Check sheet for the modelled part. Datum: model origin and axes. Units: mm. Give positions to 0.01 mm unless a question says otherwise; leave off trailing zeros. Write each loop counter-clockwise with the first axis right and the second up, starting at its lowest first coordinate (ties: lowest second). Pieces come first, ordered by that corner, then holes. Notation, with made-up numbers: (51.5, 80) -> (98.5, 80) arc R24 cw to (98.5, 104) -> close; hole circle Ø9 at (57, 17.25). An arc over 180 degrees is marked (long way). Return JSON: item names as keys, results as strings.
from build123d import *

# Parameters (mm, degrees)
BOSS_EXTRUDE1_DEPTH = 10
SKETCH2_W           = 40.182856857
SKETCH2_H           = 10
BOSS_EXTRUDE2_DEPTH = 10


with BuildPart() as part:
    # Sketch1 → Boss-Extrude1 (new body)
    with BuildSketch(Plane(origin=(0, 0, 0), x_dir=(1, 0, 0), z_dir=(0, 1, 0))):
        with BuildLine():
            Line((137, 124), (0, 124))
            Line((0, 124), (0, 0))
            Line((0, 0), (137, 0))
            Line((137, 0), (137, 12))
            Line((137, 12), (111.1, 12))
            ThreePointArc((111.1, 12), (59.1, 64), (111.1, 116))
            Line((111.1, 116), (137, 116))
            Line((137, 116), (137, 124))
        make_face()
    extrude(amount=BOSS_EXTRUDE1_DEPTH)

    # Sketch2 → Boss-Extrude2 (add)
    with BuildSketch(Plane(origin=(0, 10, 0), x_dir=(1, 0, 0), z_dir=(0, 1, 0))):
        with Locations((116.908571572, 119)):
            Rectangle(SKETCH2_W, SKETCH2_H)
    extrude(amount=-BOSS_EXTRUDE2_DEPTH)


solid = part.part
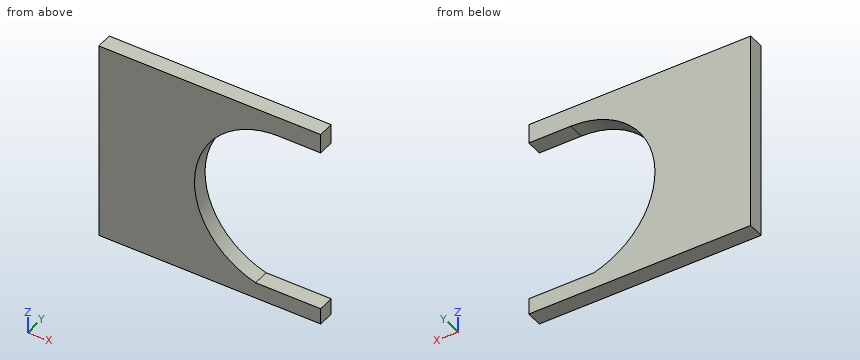
(1) Cross-section at C-C on x = 89. Enter the section's corners in (y, z).
Reply:
{"outline": "(0, -124) -> (10, -124) -> (10, -111.07) -> (0, -111.07) -> close; (0, -16.93) -> (10, -16.93) -> (10, 0) -> (0, 0) -> close"}
(2) Cross-section at D-D on z = -105.5. Enter the section's corners in (x, y), then the cut area to 3 significant figures.
Reply:
{"outline": "(0, 0) -> (79.77, 0) -> (79.77, 10) -> (0, 10) -> close", "area": "798 mm^2"}
(3) Cross-section at A-A on x = 121. Enter the section's corners in (y, z), then the cut area to 3 significant figures.
Reply:
{"outline": "(0, -124) -> (10, -124) -> (10, -114) -> (0, -114) -> close; (0, -12) -> (10, -12) -> (10, 0) -> (0, 0) -> close", "area": "220 mm^2"}
(4) Cross-section at B-B on y = 6.5. Enter the section's corners in (x, z).
Reply:
{"outline": "(0, -124) -> (137, -124) -> (137, -114) -> (96.82, -114) arc R52 cw to (111.1, -12) -> (137, -12) -> (137, 0) -> (0, 0) -> close"}
(5) Depth check by flat-ended pin: pin 1 Ø6 at (y, z) = (7.5, -56) entering from +X; pin 2 Ø4 at (y, z) = (3, -39) entering from +X; pin 3 Ø6 at (y, z) = (7, -108) entering from +X. Enter the tip coordinate at first touch or a pass-through.
Reply:
{"pin 1": "x = 60.28", "pin 2": "x = 66.66", "pin 3": "x = 88.85"}
(6) Thickness scan on L1, parallel to Z at x = 116.5, y = 5.5; L2, parallel to Z at x = 80.5, y = 7.25; L3, parallel to X at y = 8.25, z = -111.5. Record the ranges inside material, lowest first.
Reply:
{"L1": "-124 to -114, -12 to 0", "L2": "-124 to -106.04, -21.96 to 0", "L3": "0 to 89.94"}
